from build123d import *

# Parameters (mm, degrees)
SKETCH1_W           = 65.6
SKETCH1_H           = 40
BOSS_EXTRUDE1_DEPTH = 2
SKETCH2_R           = 1.5
CUT_EXTRUDE1_DEPTH  = 3
SKETCH3_W           = 35
SKETCH3_H           = 20
BOSS_EXTRUDE2_DEPTH = 4
SKETCH4_W           = 6
SKETCH4_H           = 12
BOSS_EXTRUDE3_DEPTH = 10


with BuildPart() as part:
    # Sketch1 → Boss-Extrude1 (new body)
    with BuildSketch(Plane(origin=(0, 0, 0), x_dir=(1, 0, 0), z_dir=(0, 1, 0))):
        Rectangle(SKETCH1_W, SKETCH1_H)
    extrude(amount=BOSS_EXTRUDE1_DEPTH)

    # Sketch2 → Cut-Extrude1 (cut, through all)
    with BuildSketch(Plane(origin=(0, 2, 0), x_dir=(1, 0, 0), z_dir=(0, 1, 0))):
        with Locations((-29, 17)):
            Circle(SKETCH2_R)
        with Locations((29, 17)):
            Circle(SKETCH2_R)
        with Locations((29, -17)):
            Circle(SKETCH2_R)
        with Locations((-29, -17)):
            Circle(SKETCH2_R)
    extrude(amount=-CUT_EXTRUDE1_DEPTH, mode=Mode.SUBTRACT)

    # Sketch3 → Boss-Extrude2 (add)
    with BuildSketch(Plane(origin=(0, 2, 0), x_dir=(1, 0, 0), z_dir=(0, 1, 0))):
        with Locations((0, 8)):
            Rectangle(SKETCH3_W, SKETCH3_H)
    extrude(amount=BOSS_EXTRUDE2_DEPTH)

    # Sketch4 → Boss-Extrude3 (add)
    with BuildSketch(Plane(origin=(0, 2, 0), x_dir=(1, 0, 0), z_dir=(0, 1, 0))):
        with Locations((-8, -12)):
            Rectangle(SKETCH4_W, SKETCH4_H)
        with Locations((8, -12)):
            Rectangle(SKETCH4_W, SKETCH4_H)
    extrude(amount=BOSS_EXTRUDE3_DEPTH)


solid = part.part
Build history of the part. All positions in model axes, mm. A direction names the side the tool comes from. Round coordinates to 2 decimals unless told otherwise and drop trailing zeros. Loops run counter-clockwise (first coordinate to the right, second up) from the corner with the lowest first, then second, coordinate; pieces in that order, holes last. Notation, with made-up numbers: (49.5, -14.75) -> (53.5, -14.75) arc R17 ccw to (53.5, -0.75) -> close; hole circle Ø4 at (83.25, -9). An arc over 180 degrees is marked (long way). One line per item, written item: value. Start each with the question number.
Q1. Probe line 1 along Z through (x, y) = (29, 1.45); line 2 along X through (y, z) = (1.3, -17); line 3 along X through (y, z) = (3.5, 11.5). List the from-to ranges inside material, lowest first.
Q2. Cut at A-A on z = -17. List the corners of the cut face in (x, y).
Q3. Two-plate mould, pull along Z, no slides. Class faces 1 (the face through (8, 7, 6)), 2 (the face through (32.8, 1, 0)), 3 (the face through (-8, 7, 18)): released by +Z, released by -Z, zero draft, split by the parting line, or undercut.
Q4. Cut at B-B on y = 8. List the corners of the cut face in (x, z).
Q5. Drop flat-ended pins along their axis: pin 1 Ø3 at (y, z) = (4.5, -9) entering from -X; pin 2 Ø5 at (x, y) = (-8, 9.5) entering from -Z; pin 3 Ø3.5 at (x, z) = (29, -17) entering from +Y. Give the stop position or say it passes through.
Q6. Cut at D-D on z = 12. List the corners of the cut face in (x, y).
Q7. Cut at C-C on x = 29. List the corners of the cut face in (y, z).
Q8. 3-axis set-ups, long thin cutter, end or side, ignore diameter. For faces 4 (the face through (17.5, 4, -8)), 5 (the face through (-5, 7, 12)), 6 (the face through (0, 4, 2)), 7 (the face through (0, 4, -18)), 8 (the face through (-17.5, 4, -8)): which of +Z, -Z, +X, -X, +Y, -Y reach the whole face in a straight line?
Computed:
1. line 1: -20 to -18.5, -15.5 to 15.5, 18.5 to 20
1. line 2: -32.8 to -30.5, -27.5 to 27.5, 30.5 to 32.8
1. line 3: -11 to -5, 5 to 11
2. outline: (-32.8, 0) -> (-30.5, 0) -> (-30.5, 2) -> (-32.8, 2) -> close; (-27.5, 0) -> (27.5, 0) -> (27.5, 2) -> (17.5, 2) -> (17.5, 6) -> (-17.5, 6) -> (-17.5, 2) -> (-27.5, 2) -> close; (30.5, 0) -> (32.8, 0) -> (32.8, 2) -> (30.5, 2) -> close
3. face 1: undercut
3. face 2: zero draft
3. face 3: released by +Z
4. outline: (-11, 6) -> (-5, 6) -> (-5, 18) -> (-11, 18) -> close; (5, 6) -> (11, 6) -> (11, 18) -> (5, 18) -> close
5. pin 1: x = -17.5
5. pin 2: z = 6
5. pin 3: y = 2
6. outline: (-32.8, 0) -> (32.8, 0) -> (32.8, 2) -> (11, 2) -> (11, 12) -> (5, 12) -> (5, 2) -> (-5, 2) -> (-5, 12) -> (-11, 12) -> (-11, 2) -> (-32.8, 2) -> close
7. outline: (0, -20) -> (2, -20) -> (2, -18.5) -> (0, -18.5) -> close; (0, -15.5) -> (2, -15.5) -> (2, 15.5) -> (0, 15.5) -> close; (0, 18.5) -> (2, 18.5) -> (2, 20) -> (0, 20) -> close
8. face 4: +Z, -Z, +X, +Y
8. face 5: +Z, +Y
8. face 6: +X, -X, +Y
8. face 7: -Z, +X, -X, +Y
8. face 8: +Z, -Z, -X, +Y
